Can you work these out from the model? Positions are in its coordinate system, mm. Face numbers are marked on the shaded views. Give positions to 0.01 mm unless a question says otherwise; leave off trailing zeros. Order: outer loops, then holes, each group sorted by start corner. A loop starts at its lowest first (then second) coordinate and runs counter-clockwise, first axis right, second up.
Item 1: I want a section at A-A, the plane z = 25.5. Write out the boundary of the cut face in (x, y) (3 decimals), then the cut area to 3 significant figures.
Item 2: I want a section at D-D, the plane y = 1. Count the separate pieces of the cut face and the enclosed holes in it, then the cut area to 3 significant figures.
Item 3: If I drill on line 1 along Z through (x, y) = (-6, 1); line 2 along Z through (x, y) = (0.75, 2.75); line 3 along X through (y, z) = (3.5, 29), over which ranges is the centre line in solid material (lowest first)?
Item 4: I'm going to push flat-ended pins straight in: pin 1 Ø1.5 at (y, z) = (5, 3.5) entering from -X; pin 2 Ø3 at (x, y) = (-10, 5.5) entering from +Z; pin 3 Ø3 at (y, z) = (3.5, 0) entering from +X. Where does each tip first touch, or does it pass through?
Item 5: I want a section at C-C, the plane z = 20. Write out the boundary of the cut face in (x, y), then the cut area to 3 significant figures.
Item 6: If we mould it in two halves opening along Z, with no side actions, what happens to the marked faces 1, 2 and 3? For each: +Z half, -Z half, draft (parallel to the pull), parting line (faces both ways), or undercut.
Item 7: I want a section at B-B, the plane x = -10.5. Write out the boundary of the cut face in (y, z), then the cut area to 3 significant figures.
```python
from build123d import *

# Parameters (mm, degrees)
SKETCH1_R               = 0.75
BOSS_EXTRUDE1_DEPTH     = 6.35
SKETCH2_R               = 4
SKETCH2_R_2             = 1.5
BOSS_EXTRUDE2_DEPTH     = 6.35
FILLET1_R               = 5
CUT_EXTRUDE1_DEPTH      = 36.18011987
CUT_EXTRUDE1_DEPTH_BACK = 36.18011987
FILLET2_R               = 4.5
CUT_EXTRUDE2_DEPTH      = 35.797952793
CUT_EXTRUDE2_DEPTH_BACK = 35.797952793
SKETCH5_R               = 0.75


with BuildPart() as part:
    # Sketch1 → Boss-Extrude1 (new body)
    with BuildSketch(Plane(origin=(0, 0, 0), x_dir=(1, 0, 0), z_dir=(0, 1, 0))):
        with BuildLine():
            ThreePointArc((0, 0), (-9.156655288, -11.933185502), (0, -23.866371003))
            ThreePointArc((0, -23.866371003), (2.24506403, -27.75493597), (-1.643500936, -30))
            ThreePointArc((-1.643500936, -30), (-15.506655288, -11.933185502), (-1.643500936, 6.133628997))
            ThreePointArc((-1.643500936, 6.133628997), (2.24506403, 3.888564967), (0, 0))
        make_face()
        with Locations(Location((-0.821750468, 3.066814498, 0), (0, 0, 270))):
            Circle(SKETCH1_R, mode=Mode.SUBTRACT)
        with Locations(Location((-0.821750468, -26.933185502, 0), (0, 0, 270))):
            Circle(SKETCH1_R, mode=Mode.SUBTRACT)
    extrude(amount=BOSS_EXTRUDE1_DEPTH)

    # Sketch2 → Boss-Extrude2 (add)
    # profile 1 of 2: a face of its own
    with BuildSketch(Plane(origin=(0, 6.35, 0), x_dir=(1, 0, 0), z_dir=(0, 1, 0))):
        with Locations((-0.821750468, 3.066814498)):
            Circle(SKETCH2_R)
        with Locations((-0.821750468, 3.066814498)):
            Circle(SKETCH2_R_2, mode=Mode.SUBTRACT)
    # profile 2 of 2: a face of its own
    with BuildSketch(Plane(origin=(0, 6.35, 0), x_dir=(1, 0, 0), z_dir=(0, 1, 0))):
        with Locations((-0.821750468, -26.933185502)):
            Circle(SKETCH2_R)
        with Locations((-0.821750468, -26.933185502)):
            Circle(SKETCH2_R_2, mode=Mode.SUBTRACT)
    extrude(amount=-BOSS_EXTRUDE2_DEPTH)

    # Fillet1
    fillet1_edges = [part.edges().sort_by_distance(p)[0] for p in [
        (-2.038682942, 3.175, 0.743575948),
        (-4.166745827, 3.175, -5.260215066),
        (-2.038682942, 3.175, 23.122795055),
        (-4.166745827, 3.175, 29.126586069),
    ]]
    fillet(fillet1_edges, radius=FILLET1_R)

    # Sketch4 → Cut-Extrude1 (cut, two sides: drawn at the far end of the back side and taken through both)
    with BuildSketch(Plane(origin=(0, 6.35, 0), x_dir=(1, 0, 0), z_dir=(0, 1, 0)).offset(-CUT_EXTRUDE1_DEPTH_BACK)):
        with BuildLine():
            Line((-7.783274695, -0.952423388), (-10.028338726, 1.292640642))
            ThreePointArc((-10.028338726, 1.292640642), (-14.082887201, -4.775419971), (-15.506655288, -11.933185502))
            Line((-15.506655288, -11.933185502), (-12.331655288, -11.933185502))
            ThreePointArc((-12.331655288, -11.933185502), (-11.149569685, -5.990439869), (-7.783274695, -0.952423388))
        make_face()
    extrude(amount=CUT_EXTRUDE1_DEPTH + CUT_EXTRUDE1_DEPTH_BACK, mode=Mode.SUBTRACT)

    # Chamfer1
    # the kernel refuses this chamfer: 3.25 mm, written as the material it takes off along each edge
    with BuildSketch(Plane(origin=(-15.506655288, -10.121546279, 11.933185502), x_dir=(0.9996220644729643, 0, -0.02749051143228412), z_dir=(0, 1, 0))) as chamfer1_piece_1_section:
        with BuildLine():
            Line((3.678679732, 0), (0.225552245, -4.042330768))
            Line((0.225552245, -4.042330768), (0.161654076, -4.054248153))
            ThreePointArc((0.161654076, -4.054248153), (-0.010664321, -2.031175025), (-0.064975434, 0.001786883))
            Line((-0.064975434, 0.001786883), (0.001786883, 0.064975434))
            ThreePointArc((0.001786883, 0.064975434), (1.839736708, 0.014430151), (3.680466615, 0.064975434))
            Line((3.680466615, 0.064975434), (3.678679732, 0))
        make_face()
    chamfer1_piece_1 = extrude(amount=26.593092558, mode=Mode.PRIVATE)
    chamfer1_piece_1 = chamfer1_piece_1 - Plane(origin=(3.197487418, 3.175, 11.933185502), x_dir=(-1, 0, 0), z_dir=(0, -1, 0)) * Cylinder(15.529142706, 70, mode=Mode.PRIVATE)
    add(chamfer1_piece_1, mode=Mode.SUBTRACT)
    with BuildSketch(Plane(origin=(-10.028338726, -10.121546279, -1.292640642), x_dir=(0.7634460432280789, 0, -0.6458716119163239), z_dir=(0, 1, 0))) as chamfer1_piece_2_section:
        with BuildLine():
            Line((4.048618512, 0), (0.204942617, -3.672966525))
            Line((0.204942617, -3.672966525), (0.140167642, -3.678370474))
            ThreePointArc((0.140167642, -3.678370474), (0.088085677, -1.837683405), (-0.064774975, -0.005403949))
            Line((-0.064774975, -0.005403949), (-0.005403949, 0.064774975))
            ThreePointArc((-0.005403949, 0.064774975), (2.027426371, 0.123806379), (4.056957562, 0.064462859))
            Line((4.056957562, 0.064462859), (4.048618512, 0))
        make_face()
    chamfer1_piece_2 = extrude(amount=26.593092558, mode=Mode.PRIVATE)
    chamfer1_piece_2 = chamfer1_piece_2 - Plane(origin=(3.197487418, 3.175, 11.933185502), x_dir=(-1, 0, 0), z_dir=(0, -1, 0)) * Cylinder(15.529142706, 70, mode=Mode.PRIVATE)
    add(chamfer1_piece_2, mode=Mode.SUBTRACT)

    # Fillet2
    fillet2_edges = [part.edges().sort_by_distance(p)[0] for p in [
        (-7.416497134, 3.175, 0.597507087),
        (-12.32326811, 3.175, 12.443500126),
        (-6.951183486, 3.175, -3.778257247),
        (-15.088374308, 3.175, 15.866659195),
    ]]
    fillet(fillet2_edges, radius=FILLET2_R)

    # Sketch5 → Cut-Extrude2 (cut, two sides: drawn at the far end of the back side and taken through both)
    with BuildSketch(Plane.XY.offset(-CUT_EXTRUDE2_DEPTH_BACK)):
        with Locations((-0.821750468, 3.175)):
            Circle(SKETCH5_R)
    extrude(amount=CUT_EXTRUDE2_DEPTH + CUT_EXTRUDE2_DEPTH_BACK, mode=Mode.SUBTRACT)


solid = part.part
```
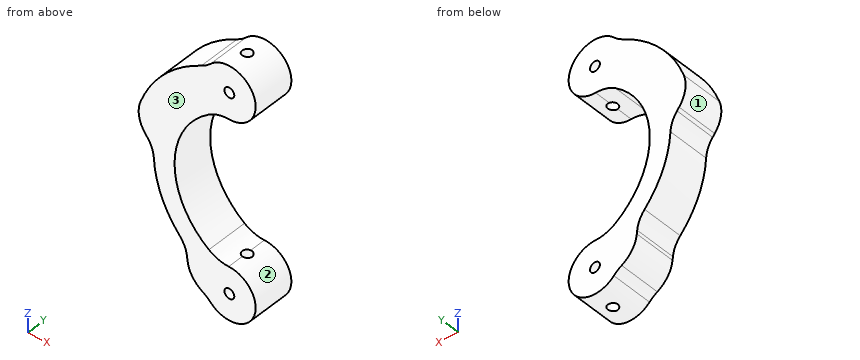
Results list:
1. outline: (-9.678, 0) - (2.913, 0) - (2.913, 6.35) - (-9.678, 6.35) - close; hole circle Ø1.5 at (-0.822, 3.175)
1. area: 78.2 mm2
2. separate pieces: 1
2. enclosed holes: 2
2. area: 253 mm2
3. line 1: z = -4.08 to 3.69, 20.18 to 28.22
3. line 2: z = -6.75 to 0.61, 23.25 to 30.61
3. line 3: x = -4.56 to -1.5, -0.15 to 2.6
4. pin 1: stops at x = -10.3
4. pin 2: stops at z = 26.53
4. pin 3: stops at x = 2.86
5. outline: (-13.68, 0) - (-6.16, 0) - (-6.16, 6.35) - (-13.68, 6.35) - close
5. area: 47.7 mm2
6. face 1: parting line
6. face 2: undercut
6. face 3: draft
7. outline: (0, 4.62) - (6.35, 4.62) - (6.35, 24.67) - (0, 24.67) - close
7. area: 127 mm2
